from build123d import *

# Parameters (mm, degrees)
BASE_FLANGE1_DEPTH = 0.8
SKETCH6_R          = 35.00000000000004
CUT_EXTRUDE1_DEPTH = 10
CUT_EXTRUDE2_DEPTH = 10
FILLET1_R          = 1
FILLET2_R          = 1
FILLET5_R          = 1
EDGE_FLANGE1_DEPTH = 549.0202041028867


# Sheet-metal steps are written as plain solids
with BuildPart() as part:
    # Base-Flange1: sheet metal written as solids
    # Sketch1 → Base-Flange1 (new body)
    with BuildSketch(Plane(origin=(0, 0, 0), x_dir=(0, 0, -1), z_dir=(1, 0, 0))):
        Polygon((-275.00000000000006, 10.101383653592132), (-82.96531829613122, 44.999999999999964), (274.99999999999994, 45.00000000000006), (274.99999999999994, -44.99999999999994), (-275.00000000000006, -45), align=None)
    extrude(amount=-BASE_FLANGE1_DEPTH)

    # Sketch6 → Cut-Extrude1 (cut)
    with BuildSketch(Plane(origin=(0, 0, 0), x_dir=(0, 0, -1), z_dir=(1, 0, 0))):
        with Locations((226.99999999999997, 0)):
            Circle(SKETCH6_R)
    extrude(amount=-CUT_EXTRUDE1_DEPTH, mode=Mode.SUBTRACT)

    # Sketch7 → Cut-Extrude2 (cut)
    with BuildSketch(Plane(origin=(0, 0, 0), x_dir=(0, 0, -1), z_dir=(1, 0, 0))):
        with BuildLine():
            Line((274.99999999999994, 45.00000000000006), (239.99999999999997, 45.00000000000006))
            ThreePointArc((239.99999999999997, 45.00000000000006), (264.74873734152914, 34.74873734152919), (274.99999999999994, 10.00000000000005))
            Line((274.99999999999994, 10.00000000000005), (274.99999999999994, 45.00000000000006))
        make_face()
    extrude(amount=-CUT_EXTRUDE2_DEPTH, mode=Mode.SUBTRACT)

    # Fillet1
    # the kernel refuses this fillet: 1 mm, written as the material it takes off along each edge
    with BuildSketch(Plane(origin=(0, 9.663409461677158, 277.4100163084993), x_dir=(-1.0, -1.5331256382814002e-12, -2.7861614884612947e-13), z_dir=(0, 0.1788022151163431, -0.9838850379335429))) as fillet1_piece_1:
        with BuildLine():
            CenterArc((1.0000000000015268, -0.979795897113006), FILLET1_R, 101.53695903288988, 78.46304096719939)
            Line((1.52675e-12, -0.9797958971145642), (-0.01999999999847325, -0.9797958971145954))
            Line((-0.01999999999847325, -0.9797958971145954), (-0.02, -3.816e-14))
            Line((-0.02, -3.816e-14), (-3.116e-14, 0.01999999999999651))
            ThreePointArc((-3.116e-14, 0.01999999999999651), (0.4000000000000967, 0.0200000000006233), (0.7960000000002303, 0.01959591794225489))
            Line((0.7960000000002303, 0.01959591794225489), (0.8000000000002557, 0))
        make_face()
    extrude(amount=204.97795897114563, mode=Mode.SUBTRACT)

    # Fillet2
    # the kernel refuses this fillet: 1 mm, written as the material it takes off along each edge
    with BuildSketch(Plane(origin=(-0.8, 10.00000000000005, -274.99999999999994), x_dir=(0, 0, 1), z_dir=(0, -1, 0))) as fillet2_piece_1:
        with BuildLine():
            CenterArc((0.9797958971145704, -1), FILLET2_R, 90, 78.46304096719936)
            Line((1.25056e-12, -0.8000000000002546), (-0.01959591794098969, -0.7960000000002597))
            ThreePointArc((-0.01959591794098969, -0.7960000000002597), (-0.01999999999998181, -0.4000000000001273), (-0.01999999999998181, 0))
            Line((-0.01999999999998181, 0), (0, 0.02000000000000002))
            Line((0, 0.02000000000000002), (0.9797958971145704, 0.02000000000000002))
            Line((0.9797958971145704, 0.02000000000000002), (0.9797958971145704, 0))
        make_face()
    extrude(amount=57.44948974278642, mode=Mode.SUBTRACT)
    with BuildSketch(Plane(origin=(-0.8, 10.000000000000078, -239.99999999999997), x_dir=(0, -1.07e-15, -1), z_dir=(0, -1, 1.07e-15))) as fillet2_piece_2:
        with BuildLine():
            CenterArc((34.0202041028854, 1), FILLET2_R, 270, 78.46304096719928)
            Line((34.99999999999872, 0.800000000000253), (35.01959591794102, 0.7960000000002581))
            ThreePointArc((35.01959591794102, 0.7960000000002581), (35.01999999999995, 0.4000000000001265), (35.01999999999995, 0))
            Line((35.01999999999995, 0), (34.999999999999915, -0.02000000000000002))
            Line((34.999999999999915, -0.02000000000000002), (34.0202041028854, -0.02000000000000002))
            Line((34.0202041028854, -0.02000000000000002), (34.0202041028854, 0))
        make_face()
    revolve(axis=Axis((-0.8, 10.000000000000078, -239.99999999999997), (1, 0, 0)), revolution_arc=90.00000000000006, mode=Mode.SUBTRACT)
    with BuildSketch(Plane(origin=(-0.8, 44.999999999999964, 90.3137875244906), x_dir=(0, -1, -2.6e-16), z_dir=(0, 2.6e-16, -1))) as fillet2_piece_3:
        with BuildLine():
            CenterArc((0.9797958971145846, -1), FILLET2_R, 90, 78.46304096719959)
            Line((1.25766e-12, -0.8000000000002574), (-0.01959591794101101, -0.7960000000002625))
            ThreePointArc((-0.01959591794101101, -0.7960000000002625), (-0.02000000000000313, -0.4000000000001287), (-0.02000000000000313, 0))
            Line((-0.02000000000000313, 0), (0, 0.02000000000000002))
            Line((0, 0.02000000000000002), (0.9797958971145846, 0.02000000000000002))
            Line((0.9797958971145846, 0.02000000000000002), (0.9797958971145846, 0))
        make_face()
    extrude(amount=330.3137875244905, mode=Mode.SUBTRACT)

    # Fillet5
    # the kernel refuses this fillet: 1 mm, written as the material it takes off along each edge
    with BuildSketch(Plane(origin=(0, -47.449489742786426, 275.00000000000006), x_dir=(-1.0, 0, -1.5631940186717228e-12), z_dir=(0, 1, 0))) as fillet5_piece_1:
        with BuildLine():
            CenterArc((1.0000000000015317, -0.9797958971130072), FILLET5_R, 101.53695903289021, 78.46304096719933)
            Line((1.53161e-12, -0.9797958971145704), (0, 0))
            Line((0, 0), (0.8000000000002546, 0))
        make_face()
    extrude(amount=59.00451925564195, mode=Mode.SUBTRACT)

    # Edge-Flange1: sheet metal written as solids
    # Edge-Flange1 section (on a plane across the edge) → Edge-Flange1 (add)
    with BuildSketch(Plane(origin=(-5.59e-15, -45.800000000000004, 274.0202041028868), x_dir=(3.49e-15, 1, 1e-16), z_dir=(0, 1e-16, -1))):
        with BuildLine():
            Line((-0.8, 0.8000000000000028), (-0.8, 19.200000000000003))
            Line((-0.8, 19.200000000000003), (0, 19.200000000000003))
            Line((0, 19.200000000000003), (0, 0.8000000000000028))
            ThreePointArc((0, 0.8000000000000028), (0.23431457505076303, 0.2343145750507638), (0.8000000000000028, 2.78e-15))
            Line((0.8000000000000028, 2.78e-15), (0.8000000000000056, -0.7999999999999973))
            ThreePointArc((0.8000000000000056, -0.7999999999999973), (-0.331370849898474, -0.3313708498984752), (-0.8, 0.8000000000000028))
        make_face()
    extrude(amount=EDGE_FLANGE1_DEPTH)


solid = part.part
Geometry check sheet. Reference: the model listing, model coordinates, mm. A direction names the side the tool comes from. Give positions to 0.01 mm unless a question says otherwise; leave off trailing zeros. Loops run counter-clockwise (first coordinate to the right, second up) from the corner with the lowest first, then second, coordinate; pieces in that order, holes last. Notation, with made-up numbers: M 20.25,-37 L 37.25,-37 A26 cw 37.25,-9 Z; hole C -1.75,-18 d9. An arc over 180 degrees is marked long. Answer as a JSON object with one key per item and string values. Group by question number.
Item 1: Sectioned sample at A-A on z = -227. Record the boundary of the cut face in (x, y).
Item 2: Material ranges on L1, parallel to X at y = -30.5, z = 134; L2, parallel to Y at x = 5.25, z = 44; L3, parallel to Y at x = -0.4, z = -227, recorded low to high.
Item 3: Sectioned sample at C-C on z = -154. Record the boundary of the cut face in (x, y).
Item 4: Access from +Z, -Z, +X, -X, +Y, -Y to the whole of each face (thin tool, end or side, straight path). Record for faces 1 (the flat face through (0, 1, -4)), 2 (the flat face through (10, -46.6, 3)).
Item 5: Sectioned sample at D-D on x = 5.25. Record the boundary of the cut face in (y, z), plus the area to 3 significant figures.
Item 6: Mould release check, pull along Y, two halves, no side actions. Record for faces 3 (the cylindrical face through (-0.39, -13.41, -259.33)), 4 (the flat face through (-0.8, 0, -3)), 5 (the cylindrical face through (-0.2, 27.4, 177.7)): pulls with the +Y half, pulls with the -Y half, needs draft (parallel to the pull), parting line crosses it, or undercut.
Item 7: Sectioned sample at B-B on y = 0. Record the boundary of the cut face in (x, z).
Item 8: Gauge pin test, flat ends, axial feed: pin 1 (1 mm diameter, centred on y = -24, z = 116.5, fed in from +X); pin 2 (6 mm diameter, centred on x = 13, z = 216, fed in from +Y); pin 3 (1.3 mm diameter, centred on x = 13.5, y = -46, fed in from +Z). Record the tip position at first contact, or that the pin passes through.
Findings below:
{
 "1": {"outline": "M -0.8,-45 A1.6 ccw 0.8,-46.6 L 19.2,-46.6 L 19.2,-45.8 L 0.8,-45.8 A0.8 cw 0,-45 L 0,-35 L -0.8,-35 Z; M -0.8,35 L 0,35 L 0,45 A1 ccw -0.8,44.02 Z"},
 "2": {"L1": "-0.8 to 0", "L2": "-46.6 to -45.8", "L3": "-46.06 to -35, 35 to 44.82"},
 "3": {"outline": "M -0.8,-45 A1.6 ccw 0.8,-46.6 L 19.2,-46.6 L 19.2,-45.8 L 0.8,-45.8 A0.8 cw 0,-45 L 0,45 A1 ccw -0.8,44.02 Z"},
 "4": {"face 1": "+Z, -Z, +X, +Y", "face 2": "+Z, -Z, +X, -X, -Y"},
 "5": {"outline": "M -46.6,-275 L -45.8,-275 L -45.8,274.02 L -46.6,274.02 Z", "area": "439 mm2"},
 "6": {"face 3": "undercut", "face 4": "needs draft", "face 5": "pulls with the +Y half"},
 "7": {"outline": "M -0.8,-274.02 A1 ccw 0,-275 L 0,-262 L -0.8,-262 Z; M -0.8,-192 L 0,-192 L 0,274.02 A1 ccw -0.8,275 Z"},
 "8": {"pin 1": "x = 0", "pin 2": "y = -45.8", "pin 3": "z = 274.02"}
}
